Here's how the part is built. I have some questions about the finished solid (model axes, mm). A direction names the side the tool comes from. Round coordinates to 2 decimals unless told otherwise and drop trailing zeros. Order: outer loops, then holes, each group sorted by start corner. A loop starts at its lowest first (then second) coordinate and runs counter-clockwise, first axis right, second up. Notation, with made-up numbers: M 11,2 L 62,2 A11 ccw 62,10 Z; hole C 23,2 d2. An arc over 180 degrees is marked long. Write each question's results on one line, items separated by ' | '. Start each with the question number.
```python
from build123d import *

# Parameters (mm, degrees)
F0_W     = 40
F0_H     = 27
F0_R     = 4.75
F0_R_2   = 4
F1_DEPTH = 10
F2_DEPTH = 2
F3_R     = 2
F4_DEPTH = 8


with BuildPart() as f1:
    # F0 (on Top) → F1 (new body)
    with BuildSketch(Plane.XY):
        Rectangle(F0_W, F0_H)
        Circle(F0_R, mode=Mode.SUBTRACT)
        Circle(F0_R)
        Circle(F0_R_2, mode=Mode.SUBTRACT)
        Circle(F0_R_2)
    extrude(amount=F1_DEPTH)

    # F0 (on Top) → F2 (cut)
    with BuildSketch(Plane.XY):
        Circle(F0_R)
        Circle(F0_R_2, mode=Mode.SUBTRACT)
    extrude(amount=F2_DEPTH, mode=Mode.SUBTRACT)

    # F3
    f3_edges = [f1.edges().sort_by_distance(p)[0] for p in [
        (20, -13.5, 5),
        (20, 13.5, 5),
        (-20, 13.5, 5),
        (-20, -13.5, 5),
    ]]
    fillet(f3_edges, radius=F3_R)

    # F4 (cut): a face of the model
    f4_faces = [f1.faces().sort_by_distance(p)[0] for p in [
        (0, 0, 0),
    ]]
    extrude(f4_faces, amount=-F4_DEPTH, mode=Mode.SUBTRACT)


solid = f1.part
```
(1) If we mould it in two halves opening along X, with no side actions, what happens to faces 1 (the flat face through (0, 0, 8)), 2 (the cylindrical face through (-19.43, 12.9, 5.07)), 3 (the cylindrical face through (-0.867, -3.905, 4.958)), 4 (the flat face through (0, 0, 10))? For each: pulls with the +X half, pulls with the -X half, needs draft (parallel to the pull), parting line crosses it, or undercut.
(2) I want a section at A-A on z = 5.25. Write out the boundary of the cut face in (x, y).
(3) Please list where these lines run through material, in increasing order: line 1 (Y direction, x = 0, z = 3.3); line 2 (Y direction, x = 0, z = 1.4); line 3 (Z direction, x = -2, y = -1.5).
(4) On a 3-axis mill with a long thin cutter (end or side, diameter ignored), from which of +Z, -Z, +X, -X, +Y, -Y can I reach the whole of each face in a straight line? I mean faces 5 (the cylindrical face through (2.192, -4.214, 0.986)), 6 (the cylindrical face through (19.4, 12.93, 5.07)). Say none if no direction works.
(5) I want a section at C-C on y = 0. Write out the boundary of the cut face in (x, z), and give its area (3 significant figures).
(6) I want a section at B-B on x = 0. Write out the boundary of the cut face in (y, z).
(7) I'm going to push a flat-ended pin straight in: pin 1 Ø2.5 at (x, y) = (-1.5, -0.5) entering from -Z. Where does the tip first touch, or does it pass through?
Solutions:
1) face 1: undercut | face 2: pulls with the -X half | face 3: undercut | face 4: needs draft
2) outline: M -20,-11.5 A2 ccw -18,-13.5 L 18,-13.5 A2 ccw 20,-11.5 L 20,11.5 A2 ccw 18,13.5 L -18,13.5 A2 ccw -20,11.5 Z; hole C 0,0 d8
3) line 1: -13.5 to -4, 4 to 13.5 | line 2: -13.5 to -4.75, 4.75 to 13.5 | line 3: 8 to 10
4) face 5: -Z | face 6: +Z, -Z, +X, +Y
5) outline: M -20,0 L -4.75,0 L -4.75,2 L -4,2 L -4,8 L 4,8 L 4,2 L 4.75,2 L 4.75,0 L 20,0 L 20,10 L -20,10 Z | area: 333 mm^2
6) outline: M -13.5,0 L -4.75,0 L -4.75,2 L -4,2 L -4,8 L 4,8 L 4,2 L 4.75,2 L 4.75,0 L 13.5,0 L 13.5,10 L -13.5,10 Z
7) pin 1: z = 8
